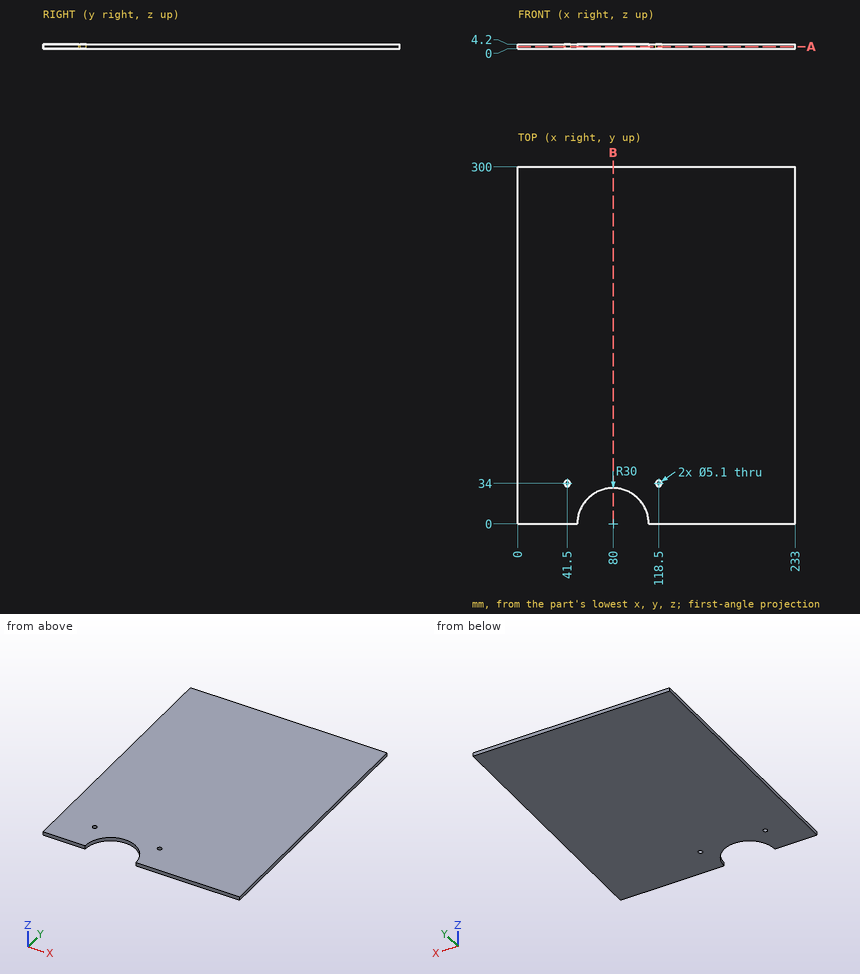
Job drawing, mm, ordinate dimensions from the low corner. One solid piece. Coordinates: 2 decimals unless noted, no trailing zeros. Order: outer loops, then holes, each group sorted by start corner. A loop starts at its lowest first (then second) coordinate and runs counter-clockwise, first axis right, second up. Notation, with made-up numbers: (-39.75, 49.5) -> (8.25, 49.5) arc R11 ccw to (8.25, 53.5) -> close; hole circle Ø11 at (83.25, 70). An arc over 180 degrees is marked (long way). Put each result on its own line as item: value. Start each with the question number.
(1) Band-saw the part on A-A (z = 1.9). Give the cut face in (x, y).
(2) Band-saw the part on B-B (x = 80). Give the cut face in (y, z), then the cut area to 3 significant figures.
(3) Probe line 1 along X through (y, z) = (34, 1.65); line 2 along Y through (x, z) = (41.5, 1.9); line 3 along Y through (x, z) = (92, 2.8). List the from-to ranges inside material, lowest first. Write a range as [from, to].
Determined:
1. outline: (0, 0) -> (50, 0) arc R30 cw to (110, 0) -> (233, 0) -> (233, 300) -> (0, 300) -> close; hole circle Ø5.1 at (41.5, 34); hole circle Ø5.1 at (118.5, 34)
2. outline: (30, 0) -> (300, 0) -> (300, 4.2) -> (30, 4.2) -> close
2. area: 1,130 mm²
3. line 1: x = [0, 38.95], [44.05, 115.95], [121.05, 233]
3. line 2: y = [0, 31.45], [36.55, 300]
3. line 3: y = [27.5, 300]
